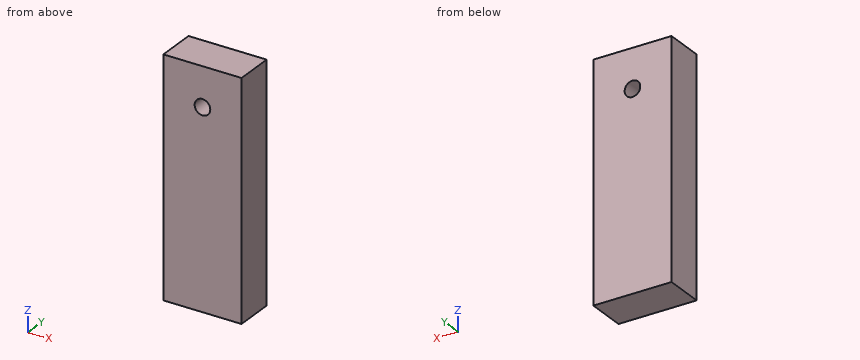
from build123d import *

# Parameters (mm, degrees)
F0_W     = 10
F0_H     = 30
F1_DEPTH = 5
F2_R     = 1
F3_DEPTH = 10


with BuildPart() as f1:
    # F0 (on Front) → F1 (new body)
    with BuildSketch(Plane.XZ):
        Rectangle(F0_W, F0_H)
    extrude(amount=F1_DEPTH)

    # F2 (on Front) → F3 (cut)
    with BuildSketch(Plane.XZ):
        with Locations((0, 10)):
            Circle(F2_R)
    extrude(amount=F3_DEPTH, mode=Mode.SUBTRACT)


solid = f1.part
Could you check a few things on this model? Use its own coordinates, in mm. Round coordinates to 2 decimals unless told otherwise and drop trailing zeros. Write each loop counter-clockwise with the first axis right and the second up, starting at its lowest first coordinate (ties: lowest second). Pieces come first, ordered by that corner, then holes. Notation, with made-up numbers: (22.5, -39) -> (58.5, -39) arc R19 cw to (58.5, -5) -> close; hole circle Ø7 at (73.25, -25). An arc over 180 degrees is marked (long way). Use a Markdown table: item, result.
1. If we section it at B-B (x = 0): List the corners of the cut face in (y, z) for me, then the cut area to 3 significant figures.
Answer key:
| item | result |
|---|---|
| outline | (-5, -15) -> (0, -15) -> (0, 9) -> (-5, 9) -> close; (-5, 11) -> (0, 11) -> (0, 15) -> (-5, 15) -> close |
| area | 140 mm^2 |
2. For pin 1 Ø1.2 at (x, z) = (0, 10) entering from +Y, with a flat end and sliding along its axis, tell me the tip position at first contact or that it passes through.
Answer key:
| item | result |
|---|---|
| pin 1 | passes through |
3. Please list where these lines run through material, in increasing order: probe 1 along X at (y, z) = (-4, 10); probe 2 along Z at (x, y) = (0, -3.4); probe 3 along Z at (x, y) = (-0.5, -1.15).
Answer key:
| item | result |
|---|---|
| probe 1 | x = -5 to -1, 1 to 5 |
| probe 2 | z = -15 to 9, 11 to 15 |
| probe 3 | z = -15 to 9.13, 10.87 to 15 |
4. If we section it at A-A (z = 10): List the corners of the cut face in (x, y) for me, then the cut area to 3 significant figures.
Answer key:
| item | result |
|---|---|
| outline | (-5, -5) -> (-1, -5) -> (-1, 0) -> (-5, 0) -> close; (1, -5) -> (5, -5) -> (5, 0) -> (1, 0) -> close |
| area | 40.0 mm^2 |
